Input: part model. Units: mm. Frame: model coordinates. Coordinates: 2 decimals unless noted, no trailing zeros. Loops run counter-clockwise (first coordinate to the right, second up) from the corner with the lowest first, then second, coordinate; pieces in that order, holes last. Notation, with made-up numbers: M -38,34.5 L -27,34.5 A27 ccw -27,60.5 Z; hole C 35,-23 d1. An arc over 180 degrees is marked long. Use a Markdown table: item, result. Add a question column.
1. Line query: L1, parallel to Y at x = 88.5, z = 1 (3 decimals); L2, parallel to Y at x = 93, z = 1 (3 decimals); L3, parallel to X at y = 45.5, z = 5.25. Output: solid intervals per line, ascending. Write a range as [from, to].
2. Section B-B on y = -9.5. Output: boundary loops of the cut face in (x, z).
3. Section C-C on z = 4.25. State how many separate pieces and enclosed holes the cut face has, then the cut area to 3 significant figures.
4. Section A-A on x = -63.5. Output: boundary loops of the cut face in (y, z).
5. Pin query (flat end, axial travel): pin 1 (1.1 mm diameter, centred on x = -73, z = 2, fed in from +Y); pin 2 (1.4 mm diameter, centred on y = -16, z = 3.5, fed in from +X); pin 3 (1.7 mm diameter, centred on y = 19, z = 3.5, fed in from +X). Return the tip coordinate at first contact, or that it passes through.
```python
from build123d import *

# Parameters (mm, degrees)
SKETCH1_W            = 203.2
SKETCH1_H            = 101.6
BOSS_EXTRUDE1_DEPTH  = 6.35
CUT_EXTRUDE2_DEPTH   = 114.769602707
MIRROR1_COPY_1_DEPTH = 114.769602707
SKETCH2_R            = 1.651
SKETCH2_W            = 44.45
SKETCH2_H            = 6.35
SKETCH2_W_2          = 38.1
CUT_EXTRUDE1_DEPTH   = 114.769602707
SKETCH4_R            = 6.35
CUT_EXTRUDE3_DEPTH   = 114.769602707
CUT_EXTRUDE4_DEPTH   = 114.769602707
LPATTERN1_COUNT      = 3
LPATTERN1_PITCH      = 9.525
CUT_EXTRUDE5_DEPTH   = 114.769602707


with BuildPart() as part:
    # Sketch1 → Boss-Extrude1 (new body)
    with BuildSketch(Plane.XY):
        Rectangle(SKETCH1_W, SKETCH1_H)
    extrude(amount=BOSS_EXTRUDE1_DEPTH)

    # Sketch3 → Cut-Extrude2 (cut, through all)
    with BuildSketch(Plane.XY.offset(6.35)):
        Polygon((101.6, 25.4), (95.25, 25.4), (95.25, 20.701), (90.17, 20.701), (90.17, 22.86), (87.63, 22.86), (87.63, 20.701), (83.82, 20.701), (83.82, 17.399), (87.63, 17.399), (87.63, 15.24), (90.17, 15.24), (90.17, 17.399), (95.25, 17.399), (95.25, 12.7), (101.6, 12.7), align=None)
    cut_extrude2 = extrude(amount=-CUT_EXTRUDE2_DEPTH, mode=Mode.SUBTRACT)

    # Mirror4: Cut-Extrude2 across plane
    add(cut_extrude2.mirror(Plane.ZX), mode=Mode.SUBTRACT)

    # Mirror1: Cut-Extrude2 across plane
    add(cut_extrude2.mirror(Plane(origin=(0, 0, 0), x_dir=(0, 0, 1), z_dir=(1, 0, 0))), mode=Mode.SUBTRACT)

    # Mirror1 copy 1 sketch → Mirror1 copy 1 (cut, through all)
    with BuildSketch(Plane(origin=(0, 0, 6.35), x_dir=(-1, 0, 0), z_dir=(0, 0, 1))):
        Polygon((101.6, 25.4), (95.25, 25.4), (95.25, 20.701), (90.17, 20.701), (90.17, 22.86), (87.63, 22.86), (87.63, 20.701), (83.82, 20.701), (83.82, 17.399), (87.63, 17.399), (87.63, 15.24), (90.17, 15.24), (90.17, 17.399), (95.25, 17.399), (95.25, 12.7), (101.6, 12.7), align=None)
    extrude(amount=-MIRROR1_COPY_1_DEPTH, mode=Mode.SUBTRACT)

    # Sketch2 → Cut-Extrude1 (cut, through all)
    with BuildSketch(Plane.XY.offset(6.35)):
        with Locations((-50.8, 47.625)):
            Circle(SKETCH2_R)
        with Locations((0, 47.625)):
            Circle(SKETCH2_R)
        with Locations((50.8, 47.625)):
            Circle(SKETCH2_R)
        with Locations((-79.375, 47.625)):
            Rectangle(SKETCH2_W, SKETCH2_H)
        with Locations((-25.4, 47.625)):
            Rectangle(SKETCH2_W_2, SKETCH2_H)
        with Locations((25.4, 47.625)):
            Rectangle(SKETCH2_W_2, SKETCH2_H)
        with Locations((79.375, 47.625)):
            Rectangle(SKETCH2_W, SKETCH2_H)
        Polygon((-57.15, -50.8), (-57.15, -41.275), (-52.451, -41.275), (-52.451, -36.195), (-54.61, -36.195), (-54.61, -33.655), (-52.451, -33.655), (-52.451, -29.845), (-49.149, -29.845), (-49.149, -33.655), (-46.99, -33.655), (-46.99, -36.195), (-49.149, -36.195), (-49.149, -41.275), (-44.45, -41.275), (-44.45, -50.8), align=None)
        Polygon((82.55, -50.8), (82.55, -41.275), (87.249, -41.275), (87.249, -36.195), (85.09, -36.195), (85.09, -33.655), (87.249, -33.655), (87.249, -29.845), (90.551, -29.845), (90.551, -33.655), (92.71, -33.655), (92.71, -36.195), (90.551, -36.195), (90.551, -41.275), (95.25, -41.275), (95.25, -50.8), align=None)
        Polygon((61.849, -29.845), (65.151, -29.845), (65.151, -43.18), (67.31, -43.18), (67.31, -45.72), (65.151, -45.72), (65.151, -50.8), (61.849, -50.8), (61.849, -45.72), (59.69, -45.72), (59.69, -43.18), (61.849, -43.18), align=None)
        Polygon((-77.851, -50.8), (-77.851, -45.72), (-80.01, -45.72), (-80.01, -43.18), (-77.851, -43.18), (-77.851, -29.845), (-74.549, -29.845), (-74.549, -43.18), (-72.39, -43.18), (-72.39, -45.72), (-74.549, -45.72), (-74.549, -50.8), align=None)
    extrude(amount=-CUT_EXTRUDE1_DEPTH, mode=Mode.SUBTRACT)

    # Sketch4 → Cut-Extrude3 (cut, through all)
    with BuildSketch(Plane.XY.offset(6.35)):
        with Locations((-63.5, 0)):
            Circle(SKETCH4_R)
    extrude(amount=-CUT_EXTRUDE3_DEPTH, mode=Mode.SUBTRACT)

    # Sketch5 → Cut-Extrude4 (cut, through all)
    with BuildSketch(Plane.XY.offset(6.35)):
        with BuildLine():
            Line((47.485508468, -34.716374897), (73.54744339, 36.888202807))
            ThreePointArc((73.54744339, 36.888202807), (77.616881416, 38.785812923), (79.514491532, 34.716374897))
            Line((79.514491532, 34.716374897), (53.45255661, -36.888202807))
            ThreePointArc((53.45255661, -36.888202807), (49.383118584, -38.785812923), (47.485508468, -34.716374897))
        make_face()
    cut_extrude4 = extrude(amount=-CUT_EXTRUDE4_DEPTH, mode=Mode.SUBTRACT)

    # LPattern1: Cut-Extrude4 ×3
    with Locations(*[(-i * LPATTERN1_PITCH, 0, 0) for i in range(1, LPATTERN1_COUNT)]):
        add(cut_extrude4, mode=Mode.SUBTRACT)

    # Sketch6 → Cut-Extrude5 (cut, through all)
    with BuildSketch(Plane.XY.offset(6.35)):
        with BuildLine():
            Line((61.952237472, -21.139086045), (74.983204933, 14.663202807))
            ThreePointArc((74.983204933, 14.663202807), (79.052642959, 16.560812923), (80.950253075, 12.491374897))
            Line((80.950253075, 12.491374897), (67.919285614, -23.310913955))
            ThreePointArc((67.919285614, -23.310913955), (63.849847588, -25.208524071), (61.952237472, -21.139086045))
        make_face()
        with BuildLine():
            Line((87.21751121, 3.540802684), (77.444285614, -23.310913955))
            ThreePointArc((77.444285614, -23.310913955), (73.374847588, -25.208524071), (71.477237472, -21.139086045))
            Line((71.477237472, -21.139086045), (81.250463068, 5.712630594))
            ThreePointArc((81.250463068, 5.712630594), (85.319901094, 7.61024071), (87.21751121, 3.540802684))
        make_face()
    extrude(amount=-CUT_EXTRUDE5_DEPTH, mode=Mode.SUBTRACT)


solid = part.part
```
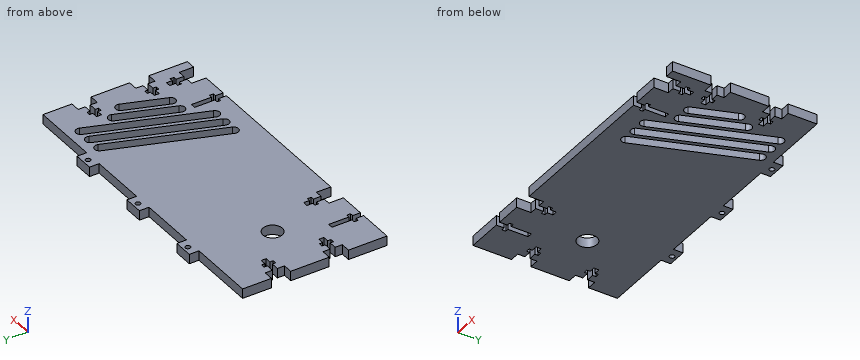
Answers below:
| question | item | result |
|---|---|---|
| 1 | L1 | y = [-29.845, -22.86], [-15.24, 15.24], [22.86, 44.45] |
| 1 | L2 | y = [-41.275, -20.701], [-17.399, 17.399], [20.701, 44.45] |
| 1 | L3 | x = [-57.15, -44.45], [-6.35, 6.35], [44.45, 57.15] |
| 2 | outline | M -101.6,0 L 37.61,0 L 37.61,6.35 L -101.6,6.35 Z; M 44.37,0 L 47.14,0 L 47.14,6.35 L 44.37,6.35 Z; M 53.9,0 L 56.66,0 L 56.66,6.35 L 53.9,6.35 Z; M 63.42,0 L 66.19,0 L 66.19,6.35 L 63.42,6.35 Z; M 72.95,0 L 75.71,0 L 75.71,6.35 L 72.95,6.35 Z; M 82.47,0 L 101.6,0 L 101.6,6.35 L 82.47,6.35 Z |
| 3 | separate pieces | 1 |
| 3 | enclosed holes | 9 |
| 3 | area | 16,400 mm² |
| 4 | outline | M -50.8,0 L -6.35,0 L -6.35,6.35 L -50.8,6.35 Z; M 6.35,0 L 44.45,0 L 44.45,6.35 L 6.35,6.35 Z |
| 5 | pin 1 | stops at y = 44.45 |
| 5 | pin 2 | stops at x = 95.25 |
| 5 | pin 3 | stops at x = 83.82 |
